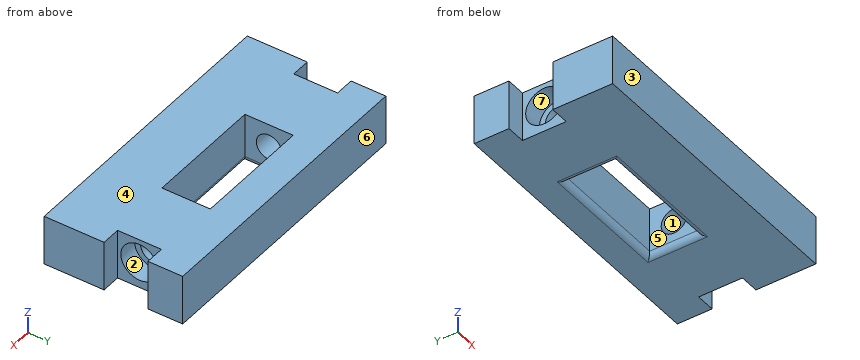
Autodesk Inventor part; units mm, degrees
ref_plane "YZ Plane" through (0, 0, 0) normal (1, 0, 0) x (0, 1, 0)
ref_plane "XZ Plane" through (0, 0, 0) normal (0, 1, 0) x (-1, 0, 0)
ref_plane "XY Plane" through (0, 0, 0) normal (0, 0, 1) x (1, 0, 0)
sketch "Sketch1" plane through (0, 0, 0) normal (0, 0, 1) x (1, 0, 0)
  line L0 (51.9, 18.35) -> (51.9, 10.6)
  line L1 (72.1, 10.6) -> (72.1, 18.35)
  line L2 (51.9, 10.6) -> (72.1, 10.6)
  line L3 (51.9, 18.35) -> (72.1, 18.35)
  line L4 (0, 21.325) -> (0, 2)
  line L5 (124, 21.325) -> (124, 2)
  line L6 (51.5, 10.2) -> (51.5, 18.75)
  line L7 (51.5, 18.75) -> (72.5, 18.75)
  line L8 (72.5, 18.75) -> (72.5, 10.2)
  line L9 (72.5, 10.2) -> (51.5, 10.2)
  line L10 (51.5, 18.35) -> (39.7, 18.35)
  line L11 (39.7, 18.35) -> (39.7, 10.6)
  line L12 (39.7, 10.6) -> (51.5, 10.6)
  line L13 (62, 18.75) -> (62, 14.7524) construction
  line L14 (72.5, 18.35) -> (84.3, 18.35)
  line L15 (84.3, 18.35) -> (84.3, 10.6)
  line L16 (84.3, 10.6) -> (72.5, 10.6)
  line L17 (36.2904, 24.5) -> (87.7096, 24.5)
  line L18 (15.65, 0) -> (108.35, 0)
  line L19 (36.2904, 24.5) -> (87.7096, 24.5)
  line L20 (87.7096, 24.5) -> (87.7096, 0)
  line L21 (87.7096, 0) -> (36.2904, 0)
  line L22 (36.2904, 0) -> (36.2904, 24.5)
  line L23 (39.7, 18.35) -> (36.2904, 18.35)
  line L24 (39.7, 10.6) -> (36.2904, 10.6)
  line L25 (84.3, 10.6) -> (87.7096, 10.6)
  line L26 (84.3, 18.35) -> (87.7096, 18.35)
  point P0 (0, 0)
  dimension "d0" = 0.4
  dimension "d1" = 11.8
extrude "Extrusion1" add sketch "Sketch1" along normal up to surface (8.8 mm away) contours L9 L8 L16 L25 L20 L18 L22 L24 L12 L6 | L12 L11 L10 L6 | L10 L23 L22 L17 L20 L26 L14 L8 L7 L6 | L8 L14 L15 L16
sketch "Sketch2" plane through (84.3, 10.6, 0) normal (1, 0, 0) x (0, 0, -1)
  circle A0 centre (-4.65, 3.875) radius 2.25
  point P0 (0, -10.6)
extrude "Extrusion2" cut sketch "Sketch2" against normal up to surface (44.6 mm away)
sketch "Sketch3" plane through (84.3, 10.6, 0) normal (1, 0, 0) x (0, 0, -1)
  circle A0 centre (-4.65, 3.875) radius 2.25
  circle A1 centre (-4.65, 3.875) radius 3.3
  point P0 (0, -10.6)
  dimension "d6" = 6.6
extrude "Extrusion3" cut sketch "Sketch3" against normal blind 3.5 contours A0 | A1
sketch "Sketch4" plane through (39.7, 10.6, 0) normal (-1, 0, 0) x (0, 0, 1)
  circle A0 centre (4.65, 3.875) radius 2.25
  circle A1 centre (4.65, 3.875) radius 3.3
  point P0 (0, -10.6)
  dimension "d9" = 6.6
extrude "Extrusion4" cut sketch "Sketch4" against normal blind 3.5 contours A0 | A1
fillet "Fillet1" radius 1 4 edges at (51.5, 14.475, 0) (72.5, 14.475, 0) (62, 18.75, 0) (62, 10.2, 0)
ref_plane "Work Plane1" through (62, 0, 39.141) normal (0, 0, -1) x (-1, 0, 0)
properties part number "Head_Baseplate"
Can you work these out from the model? Positions are in its coordinate system, mm. Face numbers are marked on the shaded views. A direction names the side the tool comes from. Round coordinates to 2 decimals unless told otherwise and drop trailing zeros. Loops run counter-clockwise (first coordinate to the right, second up) from the corner with the lowest first, then second, coordinate; pieces in that order, holes last. Notation, with made-up numbers: (-34, 20) -> (-5, 20) arc R27 cw to (-5, 55) -> close; hole circle Ø1 at (66.25, -4.75). An arc over 180 degrees is marked (long way). One line per item, written item: value. Start each with the question number.
1. If we mould it in two halves opening along Y, with no side actions, what happens to the marked faces 1, 2, 3 and 4? For each: pulls with the +Y half, pulls with the -Y half, needs draft (parallel to the pull), parting line crosses it, or undercut.
2. If we section it at D-D, the plane x = 73: Write out the boundary of the cut face in (y, z) (3 decimals), then the cut area to 3 significant figures.
3. If I drill on probe 1 along Y at (x, z) = (82.3, 4.65) (3 decimals); probe 2 along Y at (x, z) = (70, 1.75); probe 3 along X at (y, z) = (10.75, 8.25), over which ranges is the centre line in solid material (lowest first)?
4. If we section it at C-C, the plane y = 14: Write out the boundary of the cut face in (x, z).
5. For the marked faces 5, 6 and 7, which set-ups out of +Z, -Z, +X, -X, +Y, -Y let a thin tool reach every point of the face, with its end or its side?
6. If we section it at A-A, the plane x = 52: Write out the boundary of the cut face in (y, z), then the cut area to 3 significant figures.
7. For pin 1 (4 mm diameter, centred on y = 13.5, z = 6.5, fed in from +X); pin 2 (4 mm diameter, centred on y = 15, z = 6, fed in from -X); pin 3 (2.5 mm diameter, centred on y = 16, z = 4, fed in from -X), each with a flat end and sliding along its axis, tell me the tip position at first contact or that it passes through.
Calculated:
1. face 1: undercut
1. face 2: undercut
1. face 3: pulls with the -Y half
1. face 4: needs draft
2. outline: (0, 0) -> (9.2, 0) arc R1 ccw to (9.7, 0.134) -> (19.25, 0.134) arc R1 ccw to (19.75, 0) -> (24.5, 0) -> (24.5, 8.8) -> (0, 8.8) -> close; hole circle Ø4.5 at (14.475, 4.65)
2. area: 198 mm²
3. probe 1: y = 0 to 11.175, 17.775 to 24.5
3. probe 2: y = 0 to 10.2, 18.75 to 24.5
3. probe 3: x = 39.7 to 51.5, 72.5 to 84.3
4. outline: (39.7, 0) -> (50.5, 0) arc R1 ccw to (51.5, 1) -> (51.5, 2.45) -> (43.2, 2.45) -> (43.2, 1.38) -> (39.7, 1.38) -> close; (39.7, 7.92) -> (43.2, 7.92) -> (43.2, 6.85) -> (51.5, 6.85) -> (51.5, 8.8) -> (39.7, 8.8) -> close; (72.5, 1) arc R1 ccw to (73.5, 0) -> (84.3, 0) -> (84.3, 1.38) -> (80.8, 1.38) -> (80.8, 2.45) -> (72.5, 2.45) -> close; (72.5, 6.85) -> (80.8, 6.85) -> (80.8, 7.92) -> (84.3, 7.92) -> (84.3, 8.8) -> (72.5, 8.8) -> close
5. face 5: +Z, -Z
5. face 6: +Z, -Z, +X, -X, +Y
5. face 7: -X
6. outline: (0, 0) -> (9.2, 0) arc R1 ccw to (10.2, 1) -> (10.2, 8.8) -> (0, 8.8) -> close; (18.75, 1) arc R1 ccw to (19.75, 0) -> (24.5, 0) -> (24.5, 8.8) -> (18.75, 8.8) -> close
6. area: 140 mm²
7. pin 1: stops at x = 84.3
7. pin 2: stops at x = 39.7
7. pin 3: stops at x = 43.2
